Work out the finished part from the listing and answer in its coordinate system (mm). A direction names the side the tool comes from. Coordinates: 2 decimals unless noted, no trailing zeros. Loops run counter-clockwise (first coordinate to the right, second up) from the corner with the lowest first, then second, coordinate; pieces in that order, holes last. Notation, with made-up numbers: M -29.5,29 L -12.5,29 A11 ccw -12.5,36 Z; hole C -28,66 d10. An arc over 180 degrees is marked long. Write each question's results on one line, items separated by ' | '.
```python
from build123d import *

# Parameters (mm, degrees)
ESQUISSE1_W             = 580
ESQUISSE1_H             = 155
BOSS_EXTRU_1_DEPTH      = 10
ENL_V_MAT_EXTRU_1_DEPTH = 10


with BuildPart() as part:
    # Esquisse1 → Boss.-Extru.1 (new body)
    with BuildSketch(Plane(origin=(0, 0, 0), x_dir=(1, 0, 0), z_dir=(0, 1, 0))):
        with Locations((290, 77.5)):
            Rectangle(ESQUISSE1_W, ESQUISSE1_H)
    extrude(amount=BOSS_EXTRU_1_DEPTH)

    # Esquisse2 → Enlèv. mat.-Extru.1 (cut)
    with BuildSketch(Plane(origin=(0, 10, 0), x_dir=(1, 0, 0), z_dir=(0, 1, 0))):
        with BuildLine():
            Line((70, 99.405892869), (120, 99.405892869))
            ThreePointArc((120, 99.405892869), (127.071067812, 96.476960681), (130, 89.405892869))
            Line((130, 89.405892869), (130, 59.405892869))
            ThreePointArc((130, 59.405892869), (127.071067812, 52.334825057), (120, 49.405892869))
            Line((120, 49.405892869), (70, 49.405892869))
            ThreePointArc((70, 49.405892869), (62.928932188, 52.334825057), (60, 59.405892869))
            Line((60, 59.405892869), (60, 89.405892869))
            ThreePointArc((60, 89.405892869), (62.928932188, 96.476960681), (70, 99.405892869))
        make_face()
        with BuildLine():
            Line((460, 99.405892869), (510, 99.405892869))
            ThreePointArc((510, 99.405892869), (517.071067812, 96.476960681), (520, 89.405892869))
            Line((520, 89.405892869), (520, 59.405892869))
            ThreePointArc((520, 59.405892869), (517.071067812, 52.334825057), (510, 49.405892869))
            Line((510, 49.405892869), (460, 49.405892869))
            ThreePointArc((460, 49.405892869), (452.928932188, 52.334825057), (450, 59.405892869))
            Line((450, 59.405892869), (450, 89.405892869))
            ThreePointArc((450, 89.405892869), (452.928932188, 96.476960681), (460, 99.405892869))
        make_face()
    extrude(amount=-ENL_V_MAT_EXTRU_1_DEPTH, mode=Mode.SUBTRACT)


solid = part.part
```
1) Given pin 1 Ø3 at (x, z) = (306, -42.5) entering from -Y, flat-ended and moving along its own axis, determine where the tip first touches the part or whether it passes through.
Check result:
pin 1: y = 0
2) Which of the six approach directions +Z, -Z, +X, -X, +Y, -Y give full straight-line access (tool end or side, diameter ignored) to faces 1 (the face through (286, 0, -79)), 2 (the face through (60, 5, -74))?
Check result:
face 1: +Z, -Z, +X, -X, -Y | face 2: +Y, -Y
3) Straight lines are drawn through the part: probe 1 along X at (y, z) = (5.5, -81); probe 2 along Z at (x, y) = (105, 2); probe 3 along Z at (x, y) = (61.5, 9.5). For each, find the intervals that lie inside material, in ascending order. Write a range as [from, to].
Check result:
probe 1: [0, 60], [130, 450], [520, 580] | probe 2: [-155, -99.41], [-49.41, 0] | probe 3: [-155, -94.67], [-54.14, 0]
4) Find section A-A, the plane x = 79.5. Give the vertices of the cut face in (y, z).
Check result:
outline: M 0,-155 L 10,-155 L 10,-99.41 L 0,-99.41 Z; M 0,-49.41 L 10,-49.41 L 10,0 L 0,0 Z
5) Find section C-C, the plane z = -68. Give the vertices of the cut face in (x, y).
Check result:
outline: M 0,0 L 60,0 L 60,10 L 0,10 Z; M 130,0 L 450,0 L 450,10 L 130,10 Z; M 520,0 L 580,0 L 580,10 L 520,10 Z
6) For a pull along X with two mould halves and no side action, classify faces 3 (the face through (0, 5, -76)), 4 (the face through (450, 5, -74)), 5 (the face through (63.007, 5.07, -52.258)), 6 (the face through (580, 5, -76)) as released by +X, released by -X, zero draft, split by the parting line, or undercut.
Check result:
face 3: released by -X | face 4: undercut | face 5: undercut | face 6: released by +X
7) Find section B-B, the plane y = 3.75. Give the vertices of the cut face in (x, z), and give its area (3 significant figures).
Check result:
outline: M 0,-155 L 580,-155 L 580,0 L 0,0 Z; hole M 60,-89.41 A10 ccw 70,-99.41 L 120,-99.41 A10 ccw 130,-89.41 L 130,-59.41 A10 ccw 120,-49.41 L 70,-49.41 A10 ccw 60,-59.41 Z; hole M 450,-89.41 A10 ccw 460,-99.41 L 510,-99.41 A10 ccw 520,-89.41 L 520,-59.41 A10 ccw 510,-49.41 L 460,-49.41 A10 ccw 450,-59.41 Z | area: 83,100 mm^2
